from build123d import *

# Parameters (mm, degrees)
EXTRUDE1_DEPTH     = 70
SKETCH2_W          = 3
SKETCH2_H          = 3
EXTRUDE2_DEPTH     = 2.3
SKETCH3_W          = 4
SKETCH3_H          = 5
EXTRUDE3_DEPTH     = 2
SKETCH4_R          = 1
EXTRUDE4_DEPTH     = 5
FILLET1_R          = 3
SKETCH5_R          = 2.5
EXTRUDE6_DEPTH     = 5
SKETCH6_W          = 4.247308601
SKETCH6_H          = 9.124947865
CUT_EXTRUDE1_DEPTH = 10


with BuildPart() as part:
    # Sketch1 → Extrude1 (new body)
    with BuildSketch(Plane.XY):
        Polygon((-23, 9), (23, 9), (23, -9), (20.6, -9), (20.6, 6), (-23, 6), align=None)
    extrude(amount=EXTRUDE1_DEPTH)

    # Sketch2 → Extrude2 (add)
    with BuildSketch(Plane.ZY.offset(-20.6)):
        with Locations((1.5, 2.5)):
            Rectangle(SKETCH2_W, SKETCH2_H)
        with Locations((68.5, 2.5)):
            Rectangle(SKETCH2_W, SKETCH2_H)
    extrude(amount=EXTRUDE2_DEPTH)

    # Sketch3 → Extrude3 (add)
    with BuildSketch(Plane.XZ.offset(-6)):
        with Locations((-21, 8)):
            Rectangle(SKETCH3_W, SKETCH3_H)
        with Locations((-21, 62)):
            Rectangle(SKETCH3_W, SKETCH3_H)
    extrude(amount=EXTRUDE3_DEPTH)

    # Sketch4 → Extrude4 (cut)
    with BuildSketch(Plane.ZY.offset(23)):
        with Locations((8, 6.75)):
            Circle(SKETCH4_R)
        with Locations((62, 6.75)):
            Circle(SKETCH4_R)
    extrude(amount=-EXTRUDE4_DEPTH, mode=Mode.SUBTRACT)

    # Fillet1
    fillet1_edges = [part.edges().sort_by_distance(p)[0] for p in [
        (23, 9, 35),
    ]]
    fillet(fillet1_edges, radius=FILLET1_R)

    # Sketch5 → Extrude6 (cut)
    with BuildSketch(Plane(origin=(0, 9, 0), x_dir=(-1, 0, 0), z_dir=(0, 1, 0))):
        with Locations((-16.4, 9)):
            Circle(SKETCH5_R)
        with Locations((-8.9, 9)):
            Circle(SKETCH5_R)
    extrude(amount=-EXTRUDE6_DEPTH, mode=Mode.SUBTRACT)

    # Sketch6 → Cut-Extrude1 (cut)
    with BuildSketch(Plane(origin=(0, 9, 0), x_dir=(-1, 0, 0), z_dir=(0, 1, 0))):
        with Locations((19.489700301, 47.273609058)):
            Rectangle(SKETCH6_W, SKETCH6_H)
    extrude(amount=-CUT_EXTRUDE1_DEPTH, mode=Mode.SUBTRACT)


solid = part.part
Geometry check sheet. Reference: the model listing, model coordinates, mm. A direction names the side the tool comes from. Round coordinates to 2 decimals unless told otherwise and drop trailing zeros. Order: outer loops, then holes, each group sorted by start corner. A loop starts at its lowest first (then second) coordinate and runs counter-clockwise, first axis right, second up. Notation, with made-up numbers: M -28.5,-18 L 19.5,-18 A15 ccw 19.5,-1 Z; hole C -10.75,-32.5 d10. An arc over 180 degrees is marked long. Write each question's results on one line, items separated by ' | '. Start each with the question number.
1. Go/stop test with flat-tipped pins: P1, Ø8, axis at y = -0.5, z = 21, coming from the -X side; P2, Ø1, axis at x = 17.5, y = 3, coming from the -Z side; P3, Ø1, axis at x = -22, y = 5, coming from the +Z side; P4, Ø3, axis at x = -20.5, z = 62.5, coming from the -Y side. Record where each tip stops, or that it passes through.
2. Cross-section at B-B on z = 50. Record the boundary of the cut face in (x, y).
3. Cross-section at A-A on x = 8.9. Record the boundary of the cut face in (y, z), plus the area to 3 significant figures.
4. Material ranges on L1, parallel to Z at x = -21.4, y = 6.75; L2, parallel to Y at x = -21.3, z = 8; L3, parallel to Z at x = 8.9, y = 7.85, recorded low to high. Write a range as from..to.
5. Set-up check for faces 1 (the face through (-19, 5, 62)), 2 (the face through (18.3, 3, 68)), 3 (the face through (-19, 8, 51.836)), 4 (the face through (19, 4, 68)), 5 (the face through (-21, 5, 59.5)): record each of +Z, -Z, +X, -X, +Y, -Y from which the full face is reachable in a straight line by a thin tool's end or side.
6. Draft check along Z on faces 6 (the face through (18.3, 3, 1)), 7 (the face through (16.94, 7.52, 6.56)), 8 (the face through (-21, 5, 5.5)). Enter one of: pulls with the +Z half, pulls with the -Z half, needs draft (parallel to the pull), parting line crosses it, or undercut.
7. Cross-section at C-C on z = 23.5. Record the boundary of the cut face in (x, y), plus the area to 3 significant figures.
8. Cross-section at D-D on y = 6.75. Record the boundary of the cut face in (x, z).
Resolved:
1) P1: x = 20.6 | P2: through | P3: z = 64.5 | P4: y = 4
2) outline: M -23,6 L -21.61,6 L -21.61,9 L -23,9 Z; M -17.37,6 L 20.6,6 L 20.6,-9 L 23,-9 L 23,6 A3 ccw 20,9 L -17.37,9 Z
3) outline: M 6,0 L 9,0 L 9,6.5 L 6,6.5 Z; M 6,11.5 L 9,11.5 L 9,70 L 6,70 Z | area: 195 mm2
4) L1: 0..7, 9..42.71, 51.84..61, 63..70 | L2: 4..5.75, 7.75..9 | L3: 0..6.5, 11.5..70
5) face 1: +Z, -Z, -Y | face 2: +Z, -Z, -X, -Y | face 3: +Y, -Y | face 4: +Z, -Z, -X | face 5: -X, -Y
6) face 6: needs draft | face 7: undercut | face 8: pulls with the -Z half
7) outline: M -23,6 L 20.6,6 L 20.6,-9 L 23,-9 L 23,6 A3 ccw 20,9 L -23,9 Z | area: 172 mm2
8) outline: M -23,0 L 22.9,0 L 22.9,70 L -23,70 L -23,63 L -18,63 L -18,61 L -23,61 L -23,9 L -18,9 L -18,7 L -23,7 Z; hole M -21.61,42.71 L -17.37,42.71 L -17.37,51.84 L -21.61,51.84 Z; hole C 8.9,9 d5; hole C 16.4,9 d5
